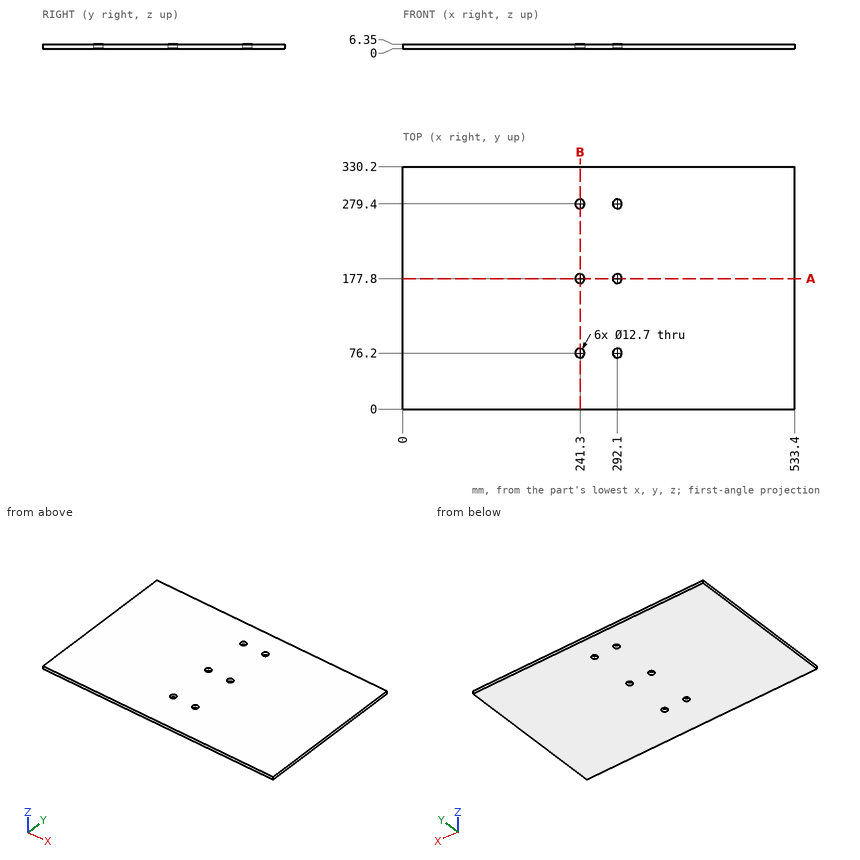
Here's the drawing with two shaded views (mm, measured from the low corner). I have some questions. Give positions to 0.01 mm unless a question says otherwise; leave off trailing zeros. Loops run counter-clockwise (first coordinate to the right, second up) from the corner with the lowest first, then second, coordinate; pieces in that order, holes last. Notation, with made-up numbers: (80.25, 71.25) -> (106.25, 71.25) arc R4 ccw to (106.25, 78.25) -> close; hole circle Ø6 at (54, 86). An arc over 180 degrees is marked (long way). Use one line per item in the form item = value.
1) If we section it at B-B (x = 241.3): Please give me the cut outline in (y, z).
Answers:
outline = (0, 0) -> (69.85, 0) -> (69.85, 6.35) -> (0, 6.35) -> close; (82.55, 0) -> (171.45, 0) -> (171.45, 6.35) -> (82.55, 6.35) -> close; (184.15, 0) -> (273.05, 0) -> (273.05, 6.35) -> (184.15, 6.35) -> close; (285.75, 0) -> (330.2, 0) -> (330.2, 6.35) -> (285.75, 6.35) -> close
2) If we section it at A-A (y = 177.8): Please give me the cut outline in (x, z), plus the area to 3 significant figures.
Answers:
outline = (0, 0) -> (234.95, 0) -> (234.95, 6.35) -> (0, 6.35) -> close; (247.65, 0) -> (285.75, 0) -> (285.75, 6.35) -> (247.65, 6.35) -> close; (298.45, 0) -> (533.4, 0) -> (533.4, 6.35) -> (298.45, 6.35) -> close
area = 3,230 mm²
3) I need wall thicknesses on line 1 along Y through (x, z) = (292.1, 1.75); line 2 along X through (y, z) = (75, 0.75); line 3 along X through (y, z) = (174, 1.5). Which ranges of each line are inside material? Lowest first, please.
Answers:
line_1 = 0 to 69.85, 82.55 to 171.45, 184.15 to 273.05, 285.75 to 330.2
line_2 = 0 to 235.06, 247.54 to 285.86, 298.34 to 533.4
line_3 = 0 to 236.21, 246.39 to 287.01, 297.19 to 533.4
4) Will this pin go through, and if not, where does the flat tip stop? pin 1 (7.5 mm diameter, centred on x = 241.3, y = 177.8, fed in from +Z).
Answers:
pin_1 = through
